```python
from build123d import *

# Parameters (mm, degrees)
SKETCH1_W           = 83
SKETCH1_H           = 53
BOSS_EXTRUDE1_DEPTH = 9
SKETCH2_W           = 83
SKETCH2_H           = 2
CUT_EXTRUDE1_DEPTH  = 2.54


with BuildPart() as part:
    # Sketch1 → Boss-Extrude1 (new body)
    with BuildSketch(Plane(origin=(0, 0, 0), x_dir=(1, 0, 0), z_dir=(0, 1, 0))):
        with Locations((41.5, -26.5)):
            Rectangle(SKETCH1_W, SKETCH1_H)
    extrude(amount=BOSS_EXTRUDE1_DEPTH)

    # Sketch2 → Cut-Extrude1 (cut)
    with BuildSketch(Plane(origin=(0, 9, 0), x_dir=(1, 0, 0), z_dir=(0, 1, 0))):
        Polygon((0, -27.5), (0, -25.5), (83, -25.5), (83, -26.5), (83, -27.5), align=None)
        with Locations((41.5, -7.159340371)):
            Rectangle(SKETCH2_W, SKETCH2_H)
        with Locations((41.5, -45.840659629)):
            Rectangle(SKETCH2_W, SKETCH2_H)
    extrude(amount=-CUT_EXTRUDE1_DEPTH, mode=Mode.SUBTRACT)


solid = part.part
```
CAD build for the part. Positions are in the model's coordinates, mm. A direction names the side the tool comes from. Coordinates: 2 decimals unless noted, no trailing zeros. Order: outer loops, then holes, each group sorted by start corner. A loop starts at its lowest first (then second) coordinate and runs counter-clockwise, first axis right, second up. Notation, with made-up numbers: M -30.75,59.25 L 11.25,59.25 A25 cw 11.25,77.25 Z; hole C 69,43.25 d8. An arc over 180 degrees is marked long. Write each question's results on one line, items separated by ' | '. Start each with the question number.
Q1. Cut at A-A (y = 7.5). List the corners of the cut face in (x, z).
Q2. Pull direction Z, two halves, no side cores. Call faces 3 (the flat face through (83, 4, 27)), 4 (the flat face through (41, 4, 53)), 5 (the flat face through (42, 6.46, 26)), 6 (the flat face through (42, 8, 27.5)): +Z half, -Z half, draft (parallel to the pull), parting line (faces both ways), or undercut.
Q3. Cut at B-B (x = 54). List the corners of the cut face in (y, z), then the cut area to 3 significant figures.
Q4. Which spindle directions (+Z, -Z, +X, -X, +Y, -Y) get a long thin tool onto all of the face, cutting with end or side? Do faces 1 (the flat face through (41, 6.46, 46)), 2 (the flat face through (41, 0, 26)). Say none if no direction does.
Q5. Drill centre lines: probe 1 along Z at (x, y) = (10, 6.5); probe 2 along Y at (x, z) = (9.5, 46). Where is each one in solid material? Low to high. Write a range as from..to.
Q6. Flat gauge pin, fed straight in: P1, Ø0.6, axis at x = 58.5, z = 26.5, coming from the +Y side. Where does the tip first touch, or does it go through?
Found:
1) outline: M 0,0 L 83,0 L 83,6.16 L 0,6.16 Z; M 0,8.16 L 83,8.16 L 83,25.5 L 0,25.5 Z; M 0,27.5 L 83,27.5 L 83,44.84 L 0,44.84 Z; M 0,46.84 L 83,46.84 L 83,53 L 0,53 Z
2) face 3: draft | face 4: +Z half | face 5: undercut | face 6: undercut
3) outline: M 0,0 L 9,0 L 9,6.16 L 6.46,6.16 L 6.46,8.16 L 9,8.16 L 9,25.5 L 6.46,25.5 L 6.46,27.5 L 9,27.5 L 9,44.84 L 6.46,44.84 L 6.46,46.84 L 9,46.84 L 9,53 L 0,53 Z | area: 462 mm²
4) face 1: +X, -X, +Y | face 2: +Z, -Z, +X, -X, -Y
5) probe 1: 0..6.16, 8.16..25.5, 27.5..44.84, 46.84..53 | probe 2: 0..6.46
6) P1: y = 6.46
